The model under review builds one solid part; all positions refer to its coordinate system, in mm. A direction names the side the tool comes from. Coordinates: 2 decimals unless noted, no trailing zeros. Write each loop counter-clockwise with the first axis right and the second up, starting at its lowest first coordinate (ties: lowest second). Pieces come first, ordered by that corner, then holes.
1) Add section B-B, the plane z = 7.5. State the section outline as (x, y) points, then the cut area to 3 significant figures.
2) Mouldability with a two-part tool opening along Y and no side actions: class faces 3 (the cylindrical face through (-5.451, 0.176, 11.746)), 4 (the flat face through (-14, -4, 1)), 5 (the flat face through (-14, 4, 1)) as released by +Y, released by -Y, zero draft, split by the parting line, or undercut.
3) Add section C-C, the plane x = 0. State the section outline as (y, z) points, then the cut area to 3 significant figures.
4) Add section D-D, the plane y = -2.5. State the section outline as (x, z) points, then the cut area to 3 significant figures.
5) Machinability: for faces 1 (the flat face through (-2, -3, 11)), 2 (the flat face through (0, 0, 15.5)), which of the approach directions +Z, -Z, +X, -X, +Y, -Y give a long, thin tool a straight path to every point of the face, cutting with its end or side? Answer none if there is none.
6) For P1, Ø6.5, axis at x = -15, y = 0.5, coming from the +Z side; P2, Ø6.5, axis at y = 0, z = 7.75, coming from the -X side; P3, Ø3, axis at x = -2.5, z = 12, coming from the +Y side; P4, Ø5, axis at x = -1.5, y = -6, coming from the -Z side, all flat-tipped, find the tip position at first contact; note any pin that passes through.
7) For line 1 (Z direction, x = 6.75, y = 0); line 2 (Z direction, x = -5.25, y = 0); line 3 (Y direction, x = -5.5, z = 7.75), list the stretches that pass through material, from the lowest coordinate up.
8) Add section A-A, the plane y = 0. State the section outline as (x, z) points, then the cut area to 3 significant figures.
from build123d import *

# Parameters (mm, degrees)
SKETCH_1_R               = 9
EXTRUDE_1_DEPTH          = 15.5
SKETCH_2_W               = 10.937742252
SKETCH_2_H               = 8
EXTRUDE_2_DEPTH          = 2.8
SKETCH_3_R               = 6.45
CUT_EXTRUDE_1_DEPTH      = 10
CUT_EXTRUDE_1_DEPTH_BACK = 2
SKETCH_4_R               = 4
CUT_EXTRUDE_2_DEPTH      = 18


with BuildPart() as part:
    # Эскиз1 → Бобышка-Вытянуть1 (new body)
    with BuildSketch(Plane.XY):
        Circle(SKETCH_1_R)
    extrude(amount=EXTRUDE_1_DEPTH)

    # Эскиз2 → Бобышка-Вытянуть2 (add)
    with BuildSketch(Plane.XY):
        with Locations((-13.531128874, 0)):
            Rectangle(SKETCH_2_W, SKETCH_2_H)
    extrude(amount=EXTRUDE_2_DEPTH)

    # Эскиз3 → Вырез-Вытянуть1 (cut, two sides)
    with BuildSketch(Plane(origin=(0, 0, 0), x_dir=(0, 0, -1), z_dir=(1, 0, 0))) as cut_extrude_1_sk:
        with Locations((-7.75, 0)):
            Circle(SKETCH_3_R)
    extrude(amount=CUT_EXTRUDE_1_DEPTH, mode=Mode.SUBTRACT)
    extrude(cut_extrude_1_sk.sketch, amount=-CUT_EXTRUDE_1_DEPTH_BACK, mode=Mode.SUBTRACT)

    # Эскиз4 → Вырез-Вытянуть2 (cut, through all)
    with BuildSketch(Plane(origin=(-2, 0, 0), x_dir=(0, 0, -1), z_dir=(1, 0, 0))):
        with Locations((-7.75, 0)):
            Circle(SKETCH_4_R)
    extrude(amount=-CUT_EXTRUDE_2_DEPTH, mode=Mode.SUBTRACT)


solid = part.part
Geometry results:
1. outline: (-8.07, -3.99) arc R9 ccw to (6.28, -6.45) - (-2, -6.45) - (-2, -3.99) - close; (-8.07, 3.99) - (-2, 3.99) - (-2, 6.45) - (6.28, 6.45) arc R9 ccw to start
1. area: 70.1 mm2
2. face 3: undercut
2. face 4: released by -Y
2. face 5: released by +Y
3. outline: (-9, 0) - (9, 0) - (9, 15.5) - (-9, 15.5) - close; hole circle Ø12.9 at (0, 7.75)
3. area: 148 mm2
4. outline: (-19, 0) - (8.65, 0) - (8.65, 1.8) - (-2, 1.8) - (-2, 4.63) - (-8.65, 4.63) - (-8.65, 2.8) - (-19, 2.8) - close; (-8.65, 10.87) - (-2, 10.87) - (-2, 13.7) - (8.65, 13.7) - (8.65, 15.5) - (-8.65, 15.5) - close
4. area: 129 mm2
5. face 1: +X
5. face 2: +Z, +X, -X, +Y, -Y
6. P1: stops at z = 2.8
6. P2: passes through
6. P3: stops at y = 8.94
6. P4: stops at z = 0
7. line 1: z = 0 to 1.3, 14.2 to 15.5
7. line 2: z = 0 to 3.75, 11.75 to 15.5
7. line 3: y = -7.12 to -4, 4 to 7.12
8. outline: (-19, 0) - (9, 0) - (9, 1.3) - (-2, 1.3) - (-2, 3.75) - (-9, 3.75) - (-9, 2.8) - (-19, 2.8) - close; (-9, 11.75) - (-2, 11.75) - (-2, 14.2) - (9, 14.2) - (9, 15.5) - (-9, 15.5) - close
8. area: 109 mm2
